from build123d import *

# Parameters (mm, degrees)
EXTRUDE_1_DEPTH             = 10
FILLET_1_R                  = 0.3
FILLET_2_R                  = 2
HOLE_WIZARD_M41_D           = 3.3
HOLE_WIZARD_M41_CSINK_D     = 4.3
HOLE_WIZARD_M41_CSINK_ANGLE = 90


with BuildPart() as part:
    # Эскиз1 → Бобышка-Вытянуть1 (new body, symmetric)
    with BuildSketch(Plane.XY):
        with BuildLine():
            Line((-4, 0), (4, 0))
            Line((4, 0), (4, -0.8))
            Line((4, -0.8), (6, -0.8))
            Line((6, -0.8), (6, -1.6))
            ThreePointArc((6, -1.6), (4.120585945, -4.832650297), (1.5, -7.5))
            Line((1.5, -7.5), (-1.5, -7.5))
            ThreePointArc((-1.5, -7.5), (-4.120585945, -4.832650297), (-6, -1.6))
            Line((-6, -1.6), (-6, -0.8))
            Line((-6, -0.8), (-4, -0.8))
            Line((-4, -0.8), (-4, 0))
        make_face()
    extrude(amount=EXTRUDE_1_DEPTH, both=True)

    # Скругление1
    fillet_1_edges = [part.edges().sort_by_distance(p)[0] for p in [
        (6, -0.8, 0),
        (6, -1.6, 0),
        (-6, -1.6, 0),
        (-6, -0.8, 0),
        (-4, 0, 0),
        (4, 0, 0),
    ]]
    fillet(fillet_1_edges, radius=FILLET_1_R)

    # Скругление2
    fillet_2_edges = [part.edges().sort_by_distance(p)[0] for p in [
        (1.5, -7.5, 0),
        (-1.5, -7.5, 0),
    ]]
    fillet(fillet_2_edges, radius=FILLET_2_R)

    # Отверстие обработанное метчиком M41 (through all)
    with Locations(Plane(origin=(0, 0, 0), x_dir=(1, 0, 0), z_dir=(0, 1, 0))):
        with Locations((0, -4)):
            CounterSinkHole(HOLE_WIZARD_M41_D / 2, HOLE_WIZARD_M41_CSINK_D / 2, counter_sink_angle=HOLE_WIZARD_M41_CSINK_ANGLE)

    # Эскиз5 → Повернуть1 (revolve)
    with BuildSketch(Plane(origin=(0, 0, 0), x_dir=(0, 0, -1), z_dir=(1, 0, 0))):
        with BuildLine():
            Line((6, -4.3), (6, -8.3))
            ThreePointArc((6, -8.3), (4, -6.3), (6, -4.3))
        make_face()
    revolve(axis=Axis((0, -4.3, -6), (0, -1, 0)))


solid = part.part
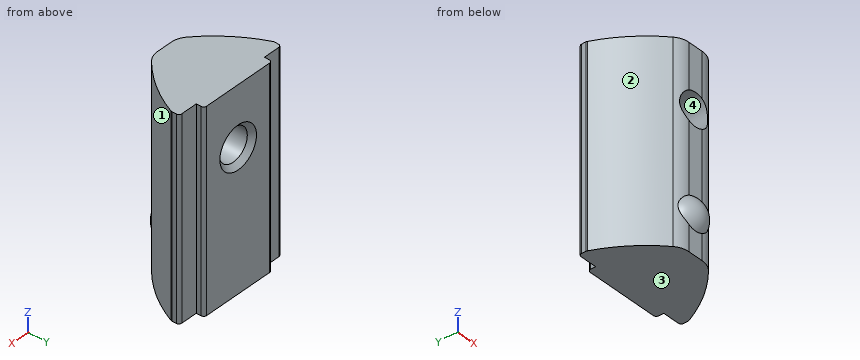
Work out the finished part from the listing and answer in its coordinate system (mm). Face numbers are marked on the shaded views. Round coordinates to 2 decimals unless told otherwise and drop trailing zeros. Order: outer loops, then holes, each group sorted by start corner. A loop starts at its lowest first (then second) coordinate and runs counter-clockwise, first axis right, second up. Notation, with made-up numbers: M 81.5,35.5 L 110.5,35.5 A26 ccw 110.5,61.5 Z; hole C -20.5,62.5 d1. An arc over 180 degrees is marked long. One line per item, written item: value.
Q1. Straight lines are drawn through the part: line 1 (Z direction, x = 0, y = -5.5); line 2 (X direction, y = -2.25, z = 4); line 3 (X direction, y = -5.25, z = 4). For each, find the intervals that lie inside material, in ascending order.
Derived:
line 1: -10 to 2.35, 5.65 to 10
line 2: -5.71 to -1.65, 1.65 to 5.71
line 3: -3.79 to -1.65, 1.65 to 3.79
Q2. Find section A-A on x = 0. Write down the section's boundary in (y, z).
Derived:
outline: M -7.5,-10 L 0,-10 L 0,1.85 L -0.5,2.35 L -7.5,2.35 L -7.5,-4.4 A2 ccw -7.5,-7.6 Z; M -7.5,5.65 L -0.5,5.65 L 0,6.15 L 0,10 L -7.5,10 Z
Q3. Flat-ended cylindrical pins translate along their axes: pin 1 (1.5 mm diameter, centred on y = -4.5, z = -5, fed in from -X); pin 2 (1 mm diameter, centred on x = 3.5, z = 1.5, fed in from -Y); pin 3 (1.4 mm diameter, centred on x = -4.5, z = 4.5, fed in from +Y). Find the tip coordinate at first contact, or state that the pin passes through.
Derived:
pin 1: x = -4.87
pin 2: y = -6.14
pin 3: y = -0.02
Q4. Find section D-D on z = -3.5. Write down the section's boundary in (x, y).
Derived:
outline: M -6,-1.54 A0.3 ccw -5.98,-1.66 A15 ccw -2.1,-7 A2 ccw -0.78,-7.5 L 0.78,-7.5 A2 ccw 2.1,-7 A15 ccw 5.98,-1.66 A0.3 ccw 6,-1.54 L 6,-1.1 A0.3 ccw 5.7,-0.8 L 4,-0.8 L 4,-0.3 A0.3 ccw 3.7,0 L -3.7,0 A0.3 ccw -4,-0.3 L -4,-0.8 L -5.7,-0.8 A0.3 ccw -6,-1.1 Z
Q5. Find section C-C on y = -3.75. Write down the section's boundary in (x, z), then the cut area to 3 significant figures.
Derived:
outline: M -4.87,-10 L 4.87,-10 L 4.87,10 L -4.87,10 Z; hole C 0,4 d3.3
area: 186 mm²
Q6. Determine the mould class of the marked faces 1, 2, 3 and 4 for opening direction X: released by +X, released by -X, zero draft, split by the parting line, or undercut.
Derived:
face 1: released by +X
face 2: released by -X
face 3: zero draft
face 4: undercut
Q7. Find section B-B on z = 4. Write down the section's boundary in (x, y).
Derived:
outline: M -6,-1.54 A0.3 ccw -5.98,-1.66 A15 ccw -2.1,-7 A2 ccw -1.65,-7.3 L -1.65,-0.5 L -2.15,0 L -3.7,0 A0.3 ccw -4,-0.3 L -4,-0.8 L -5.7,-0.8 A0.3 ccw -6,-1.1 Z; M 1.65,-7.3 A2 ccw 2.1,-7 A15 ccw 5.98,-1.66 A0.3 ccw 6,-1.54 L 6,-1.1 A0.3 ccw 5.7,-0.8 L 4,-0.8 L 4,-0.3 A0.3 ccw 3.7,0 L 2.15,0 L 1.65,-0.5 Z
